Input: part model. Units: mm. Frame: model coordinates. Face numbers are marked on the shaded views. A direction names the side the tool comes from. Round coordinates to 2 decimals unless told otherwise and drop trailing zeros. Loops run counter-clockwise (first coordinate to the right, second up) from the corner with the lowest first, then second, coordinate; pieces in that order, holes last. Notation, with made-up numbers: (78, 66.25) - (117, 66.25) arc R22 ccw to (117, 82.25) - close; hole circle Ø10 at (-7.75, 20). An arc over 180 degrees is marked (long way). Write each question's results on one line, items separated by ' | '.
Autodesk Inventor part; units mm, degrees
ref_plane "YZ Plane" through (0, 0, 0) normal (1, 0, 0) x (0, 1, 0)
ref_plane "XZ Plane" through (0, 0, 0) normal (0, 1, 0) x (-1, 0, 0)
ref_plane "XY Plane" through (0, 0, 0) normal (0, 0, 1) x (1, 0, 0)
sketch "草圖1" plane through (0, 0, 0) normal (1, 0, 0) x (0, 1, 0)
  line L0 (0, 0) -> (6.3397, 0)
  line L1 (6.3397, 0) -> (15, -5)
  line L2 (15, -5) -> (15, -16)
  line L3 (15, -16) -> (12, -20)
  line L4 (12, -20) -> (0, -20)
  line L5 (0, -20) -> (0, 0)
  dimension "d0" = 15
  dimension "d1" = 20
  dimension "d2" = 60
  dimension "d3" = 5
  dimension "d4" = 4
  dimension "d5" = 3
extrude "擠出1" add sketch "草圖1" along normal blind 8
sketch "草圖2" plane through (8, 0, 0) normal (1, 0, 0) x (0, 0, -1)
  line L0 (0, 0) -> (20, 0)
  line L1 (15, 0) -> (15, 8)
  arc A0 (15, 8) -> (5, 8) centre (10, 8) ccw
  line L2 (5, 8) -> (5, 0)
  line L3 (5, 8) -> (16.8472, 8) construction
  line L4 (10, 8) -> (10, 12.4145) construction
  line L5 (0, 6.3397) -> (0, 0)
  line L6 (5, 0) -> (15, 0)
  dimension "d8" = 10
  dimension "d9" = 5
  dimension "d10" = 8
extrude "擠出2" add sketch "草圖2" along normal blind 8
fillet "圓角1" radius 3 3 edges at (8, 13, -10) (8, 4, -15) (8, 4, -5)
sketch "草圖3" plane through (16, 0, 0) normal (1, 0, 0) x (0, 0, -1)
  arc A0 (15, 8) -> (5, 8) centre (10, 8) ccw
  circle A1 centre (10, 8) radius 2.5
  point P0 (0, 0)
  dimension "d14" = 5
extrude "擠出3" cut sketch "草圖3" against normal up to next
properties part number "410571040示範二"
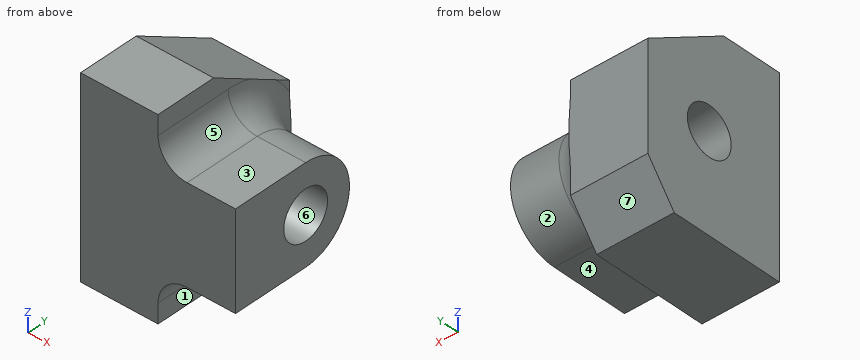
1. Section query D-D, the plane x = 14. Output: boundary loops of the cut face in (y, z).
Answer:
outline: (0, -15) - (8, -15) arc R5 ccw to (8, -5) - (0, -5) - close; hole circle Ø5 at (8, -10)
2. Section query B-B, the plane x = 3.75. Output: boundary loops of the cut face in (y, z), plus the area to 3 significant figures.
Answer:
outline: (0, -20) - (12, -20) - (15, -16) - (15, -5) - (6.34, 0) - (0, 0) - close; hole circle Ø5 at (8, -10) | area: 253 mm^2
3. Line query: line 1 (Y direction, x = 12, z = -10); line 2 (Y direction, x = 10.25, z = -10); line 3 (X direction, y = 4, z = -1.75). Output: solid intervals per line, ascending. Write a range as [from, to].
Answer:
line 1: [0, 5.5], [10.5, 13] | line 2: [0, 5.5], [10.5, 13.1] | line 3: [0, 8]
4. Section query C-C, the plane y = 2. Output: boundary loops of the cut face in (x, z), plus the area to 3 significant figures.
Answer:
outline: (0, -20) - (8, -20) - (8, -18) arc R3 cw to (11, -15) - (16, -15) - (16, -5) - (11, -5) arc R3 cw to (8, -2) - (8, 0) - (0, 0) - close | area: 244 mm^2
5. Section query A-A, the plane z = -10. Output: boundary loops of the cut face in (x, y).
Answer:
outline: (0, 0) - (16, 0) - (16, 5.5) - (0, 5.5) - close; (0, 10.5) - (16, 10.5) - (16, 13) - (11, 13) arc R3 cw to (8.17, 15) - (0, 15) - close
6. Set-up query: the marked faces 1, 2, 3 and 4. Return all of +Z, -Z, +X, -X, +Y, -Y with unobstructed straight access to the full face (end or side cutting, diameter ignored); none if empty.
Answer:
face 1: -Z, +X, +Y | face 2: +X, +Y | face 3: +Z, +X, +Y, -Y | face 4: -Z, +X, +Y, -Y
7. Contact query for flat-ended pins moving along their axis: pin 1 (1.2 mm diameter, centred on y = 3, z = -0.5, fed in from +X); pin 2 (1.8 mm diameter, centred on y = 14, z = -5.5, fed in from +X); pin 3 (5.5 mm diameter, centred on x = 12.5, y = 3.5, fed in from +Z). Output: stop coordinate, or through.
Answer:
pin 1: x = 8 | pin 2: x = 8.35 | pin 3: z = -4.73
8. Mould query, pull axis Y, two halves, no side actions, for the marked faces 5, 6 and 7. Classes: pulls with the +Y half, pulls with the -Y half, needs draft (parallel to the pull), parting line crosses it, or undercut.
Answer:
face 5: needs draft | face 6: undercut | face 7: pulls with the +Y half
